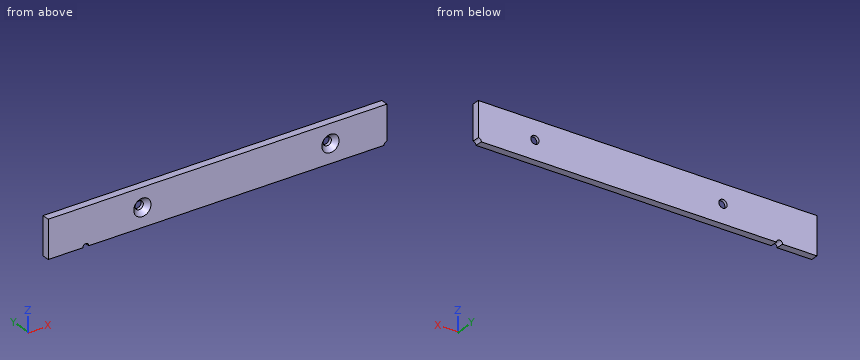
from build123d import *

# Parameters (mm, degrees)
CROQUIS1_W                                           = 226
CROQUIS1_H                                           = 25
SALIENTE_EXTRUIR1_DEPTH                              = 5
CROQUIS2_R                                           = 2
CORTAR_EXTRUIR1_DEPTH                                = 5
AVELLANADO_PARA_TORNILLO_CON_CABEZA_AVEL_D           = 5.5
AVELLANADO_PARA_TORNILLO_CON_CABEZA_AVEL_DEPTH       = 5
AVELLANADO_PARA_TORNILLO_CON_CABEZA_AVEL_CSINK_D     = 11.47
AVELLANADO_PARA_TORNILLO_CON_CABEZA_AVEL_CSINK_ANGLE = 90
AVELLANADO_PARA_TORNILLO_CON_CABEZA_AVEL_TIP         = 1.652366702


with BuildPart() as part:
    # Croquis1 → Saliente-Extruir1 (new body)
    with BuildSketch(Plane(origin=(0, 0, 0), x_dir=(1, 0, 0), z_dir=(0, 1, 0))):
        with Locations((113, 12.5)):
            Rectangle(CROQUIS1_W, CROQUIS1_H)
    extrude(amount=SALIENTE_EXTRUIR1_DEPTH)

    # Croquis2 → Cortar-Extruir1 (cut)
    with BuildSketch(Plane(origin=(0, 5, 0), x_dir=(1, 0, 0), z_dir=(0, 1, 0))):
        with Locations((25, 25)):
            Circle(CROQUIS2_R)
        with Locations((226, 25)):
            Circle(CROQUIS2_R)
    extrude(amount=-CORTAR_EXTRUIR1_DEPTH, mode=Mode.SUBTRACT)

    # Avellanado para tornillo con cabeza avellanada de clavija hexagonal de M51
    with Locations(Plane(origin=(0, 0, 0), x_dir=(-1, 0, 0), z_dir=(0, -1, 0))):
        with Locations((-62.75, 12.5), (-188.25, 12.5)):
            CounterSinkHole(AVELLANADO_PARA_TORNILLO_CON_CABEZA_AVEL_D / 2, AVELLANADO_PARA_TORNILLO_CON_CABEZA_AVEL_CSINK_D / 2, depth=AVELLANADO_PARA_TORNILLO_CON_CABEZA_AVEL_DEPTH, counter_sink_angle=AVELLANADO_PARA_TORNILLO_CON_CABEZA_AVEL_CSINK_ANGLE)
            with Locations((0, 0, -(AVELLANADO_PARA_TORNILLO_CON_CABEZA_AVEL_DEPTH + AVELLANADO_PARA_TORNILLO_CON_CABEZA_AVEL_TIP / 2))):  # 118° drill point
                Cone(0, AVELLANADO_PARA_TORNILLO_CON_CABEZA_AVEL_D / 2, AVELLANADO_PARA_TORNILLO_CON_CABEZA_AVEL_TIP, mode=Mode.SUBTRACT)


solid = part.part
Geometry check sheet. Reference: the model listing, model coordinates, mm. Give positions to 0.01 mm unless a question says otherwise; leave off trailing zeros. Write each loop counter-clockwise with the first axis right and the second up, starting at its lowest first coordinate (ties: lowest second). Pieces come first, ordered by that corner, then holes. Notation, with made-up numbers: (16.5, 86) - (20.5, 86) arc R33 cw to (20.5, 116) - close; hole circle Ø3 at (-11, 9). An arc over 180 degrees is marked (long way). Put each result on its own line as item: value.
1. Sectioned sample at B-B, the plane x = 62.75. Enter the section's corners in (y, z) (3 decimals), plus the area to 3 significant figures.
Ans:
outline: (0, -25) - (5, -25) - (5, -15.25) - (2.985, -15.25) - (0, -18.235) - close; (0, -6.765) - (2.985, -9.75) - (5, -9.75) - (5, 0) - (0, 0) - close
area: 88.6 mm²
2. Thickness scan on line 1 (Z direction, x = 188.25, y = 3.4); line 2 (X direction, y = 1.1, z = -9.25); line 3 (X direction, y = 2.6, z = -11.75). Record the ranges inside material, lowest first.
Ans:
line 1: z = -25 to -15.25, -9.75 to 0
line 2: x = 0 to 59.45, 66.05 to 184.95, 191.55 to 226
line 3: x = 0 to 59.71, 65.79 to 185.21, 191.29 to 226
3. Sectioned sample at D-D, the plane x = 25. Enter the section's corners in (y, z), plus the area to 3 significant figures.
Ans:
outline: (0, -23) - (5, -23) - (5, 0) - (0, 0) - close
area: 115 mm²
4. Sectioned sample at A-A, the plane z = -12.5. Enter the section's corners in (x, y) (3 decimals).
Ans:
outline: (0, 0) - (57.015, 0) - (60, 2.985) - (60, 5) - (0, 5) - close; (65.5, 2.985) - (68.485, 0) - (182.515, 0) - (185.5, 2.985) - (185.5, 5) - (65.5, 5) - close; (191, 2.985) - (193.985, 0) - (226, 0) - (226, 5) - (191, 5) - close
5. Sectioned sample at C-C, the plane y = 0.75. Enter the section's corners in (x, z) (3 decimals).
Ans:
outline: (0, -25) - (23, -25) arc R2 cw to (27, -25) - (224, -25) arc R2 cw to (226, -23) - (226, 0) - (0, 0) - close; hole circle Ø9.97 at (62.75, -12.5); hole circle Ø9.97 at (188.25, -12.5)
